```python
from build123d import *

# Parameters (mm, degrees)
SKETCH1_W                                = 24
SKETCH1_H                                = 5
BOSS_EXTRUDE1_DEPTH                      = 15
SKETCH2_R                                = 1.15
BOSS_EXTRUDE2_DEPTH                      = 5
SKETCH4_R                                = 4
CUT_EXTRUDE1_DEPTH                       = 11
CBORE_FOR_M3_PAN_HEAD_SCREW1_D           = 3.6
CBORE_FOR_M3_PAN_HEAD_SCREW1_CBORE_D     = 7
CBORE_FOR_M3_PAN_HEAD_SCREW1_CBORE_DEPTH = 2.4


with BuildPart() as part:
    # Sketch1 → Boss-Extrude1 (new body)
    with BuildSketch(Plane(origin=(0, 0, 0), x_dir=(0, 0, -1), z_dir=(1, 0, 0))):
        Rectangle(SKETCH1_W, SKETCH1_H)
    extrude(amount=BOSS_EXTRUDE1_DEPTH)

    # Sketch2 → Boss-Extrude2 (add)
    with BuildSketch(Plane.XZ.offset(2.5)):
        with Locations((2, 9)):
            Circle(SKETCH2_R)
        with Locations((13, 9)):
            Circle(SKETCH2_R)
        with Locations((13, -9)):
            Circle(SKETCH2_R)
        with Locations((2, -9)):
            Circle(SKETCH2_R)
    extrude(amount=BOSS_EXTRUDE2_DEPTH)

    # Sketch4 → Cut-Extrude1 (cut, through all)
    with BuildSketch(Plane(origin=(0, 2.5, 0), x_dir=(1, 0, 0), z_dir=(0, 1, 0))):
        with Locations((7.5, 0)):
            Circle(SKETCH4_R)
    extrude(amount=-CUT_EXTRUDE1_DEPTH, mode=Mode.SUBTRACT)

    # CBORE for M3 Pan Head Screw1 (through all)
    with Locations(Plane(origin=(0, -2.5, 0), x_dir=(-1, 0, 0), z_dir=(0, -1, 0))):
        with Locations((-7.5, 8), (-7.5, -8)):
            CounterBoreHole(CBORE_FOR_M3_PAN_HEAD_SCREW1_D / 2, CBORE_FOR_M3_PAN_HEAD_SCREW1_CBORE_D / 2, CBORE_FOR_M3_PAN_HEAD_SCREW1_CBORE_DEPTH)


solid = part.part
```
Work out the finished part from the listing and answer in its coordinate system (mm). A direction names the side the tool comes from. Give positions to 0.01 mm unless a question says otherwise; leave off trailing zeros. Write each loop counter-clockwise with the first axis right and the second up, starting at its lowest first coordinate (ties: lowest second). Pieces come first, ordered by that corner, then holes.
(1) Straight lines are drawn through the part: line 1 (Z direction, x = 7.5, y = 1.85); line 2 (Z direction, x = 7.5, y = -0.55); line 3 (X direction, y = 2, z = 0). For each, find the intervals that lie inside material, in ascending order.
Final values:
line 1: z = -12 to -9.8, -6.2 to -4, 4 to 6.2, 9.8 to 12
line 2: z = -12 to -11.5, -4.5 to -4, 4 to 4.5, 11.5 to 12
line 3: x = 0 to 3.5, 11.5 to 15
(2) The part is cut by section D-D on x = 10. Write down the section's boundary in (y, z), plus the area to 3 significant figures.
Final values:
outline: (-2.5, -12) - (2.5, -12) - (2.5, -3.12) - (-2.5, -3.12) - (-2.5, -5.55) - (-0.1, -5.55) - (-0.1, -10.45) - (-2.5, -10.45) - close; (-2.5, 3.12) - (2.5, 3.12) - (2.5, 12) - (-2.5, 12) - (-2.5, 10.45) - (-0.1, 10.45) - (-0.1, 5.55) - (-2.5, 5.55) - close
area: 65.3 mm2
(3) The part is cut by section B-B on x = 7.5. Write down the section's boundary in (y, z).
Final values:
outline: (-2.5, -12) - (2.5, -12) - (2.5, -9.8) - (-0.1, -9.8) - (-0.1, -11.5) - (-2.5, -11.5) - close; (-2.5, -4.5) - (-0.1, -4.5) - (-0.1, -6.2) - (2.5, -6.2) - (2.5, -4) - (-2.5, -4) - close; (-2.5, 4) - (2.5, 4) - (2.5, 6.2) - (-0.1, 6.2) - (-0.1, 4.5) - (-2.5, 4.5) - close; (-2.5, 11.5) - (-0.1, 11.5) - (-0.1, 9.8) - (2.5, 9.8) - (2.5, 12) - (-2.5, 12) - close
(4) The part is cut by section A-A on y = -2.25. Write down the section's boundary in (x, z), plus the area to 3 significant figures.
Final values:
outline: (0, -12) - (15, -12) - (15, 12) - (0, 12) - close; hole circle Ø8 at (7.5, 0); hole circle Ø7 at (7.5, -8); hole circle Ø7 at (7.5, 8)
area: 233 mm2
(5) Flat-ended cylindrical pins translate along their axes: pin 1 Ø1 at (x, z) = (8.5, -8) entering from +Y (3 decimals); pin 2 Ø6 at (x, z) = (7.5, -8) entering from +Y; pin 3 Ø2 at (x, y) = (12.5, -4) entering from -Z; pin 4 Ø2 at (x, z) = (7, -7) entering from -Y. Find the tip coordinate at first contact, or state that the pin passes through.
Final values:
pin 1: passes through
pin 2: stops at y = 2.5
pin 3: stops at z = -10.15
pin 4: stops at y = -0.1
(6) Which of the six approach directions +Z, -Z, +X, -X, +Y, -Y give full straight-line access (tool end or side, diameter ignored) to faces 1 (the cylindrical face through (7.11, 1.218, 9.757)), 2 (the flat face through (8, -0.1, 6))?
Final values:
face 1: +Y, -Y
face 2: -Y
(7) The part is cut by section C-C on z = -6.5. Write down the section's boundary in (x, y), plus the area to 3 significant figures.
Final values:
outline: (0, -2.5) - (4.34, -2.5) - (4.34, -0.1) - (6.51, -0.1) - (6.51, 2.5) - (0, 2.5) - close; (8.49, -0.1) - (10.66, -0.1) - (10.66, -2.5) - (15, -2.5) - (15, 2.5) - (8.49, 2.5) - close
area: 54.6 mm2
(8) The mould has two halves that part along X. Classify faces 3 (the flat face through (15, 0, 0)), 4 (the cylindrical face through (12.751, -4.965, 7.877)), 5 (the flat face through (4.1, 2.5, -2.5)): pulls with the +X half, pulls with the -X half, needs draft (parallel to the pull), parting line crosses it, or undercut.
Final values:
face 3: pulls with the +X half
face 4: undercut
face 5: needs draft
